Can you work these out from the model? Positions are in its coordinate system, mm. A direction names the side the tool comes from. Coordinates: 2 decimals unless noted, no trailing zeros. Loops run counter-clockwise (first coordinate to the right, second up) from the corner with the lowest first, then second, coordinate; pieces in that order, holes last.
Autodesk Inventor part; units mm, degrees
ref_plane "YZ Plane" through (0, 0, 0) normal (1, 0, 0) x (0, 1, 0)
ref_plane "XZ Plane" through (0, 0, 0) normal (0, 1, 0) x (-1, 0, 0)
ref_plane "XY Plane" through (0, 0, 0) normal (0, 0, 1) x (1, 0, 0)
sketch "スケッチ1" plane through (0, 0, 0) normal (0, 0, 1) x (1, 0, 0)
  line L0 (-12, -6) -> (12, -6)
  line L1 (12, -6) -> (12, 6)
  line L2 (12, 6) -> (-12, 6)
  line L3 (-12, 6) -> (-12, -6)
  line L4 (-12, -6) -> (12, 6) construction
  line L5 (12, -6) -> (-12, 6) construction
  point P0 (0, 0)
  dimension "d0" = 24
  dimension "d1" = 12
extrude "押し出し1" add sketch "スケッチ1" against normal blind 26.7
sketch "スケッチ2" plane through (0, 0, 0) normal (0, 0, 1) x (1, 0, 0)
  line L0 (-15, 0) -> (15, 0) construction
  line L1 (-15, -4) -> (15, -4)
  line L2 (15, 4) -> (-15, 4)
  arc A0 (-15, 4) -> (-15, -4) centre (-15, 0) ccw
  arc A1 (15, -4) -> (15, 4) centre (15, 0) ccw
  point P0 (0, 0)
  dimension "d4" = 30
  dimension "d5" = 4
extrude "押し出し2" add sketch "スケッチ2" against normal blind 7
sketch "スケッチ3" plane through (0, 0, 0) normal (0, 0, 1) x (1, 0, 0)
  arc A0 (-15, 4) -> (-15, -4) centre (-15, 0) ccw
  arc A1 (15, -4) -> (15, 4) centre (15, 0) ccw
  point P0 (0, 0)
hole "穴1" at (15, 0, 0) at (-15, 0, 0) direction (0, 0, -1) diameter 2.459 end through all
sketch "スケッチ4" plane through (0, 0, -26.7) normal (0, 0, -1) x (-1, 0, 0)
  circle A0 centre (0, 0) radius 5.5
  line L0 (12, 6) -> (-12, 6)
  dimension "d30" = 11
extrude "押し出し3" add sketch "スケッチ4" along normal blind 2.8
sketch "スケッチ5" plane through (-12, 6, 0) normal (0, 1, 0) x (1, 0, 0)
  line L0 (17.5, 29.5) -> (6.5, 29.5)
  line L1 (6.5, 26.7) -> (17.5, 26.7)
  line L2 (6.5, 26.7) -> (17.5, 26.7)
  line L3 (6.5, 26.7) -> (6.5, 26.7)
  line L4 (17.5, 26.7) -> (24, 15)
  line L5 (24, 0) -> (24, 26.7)
  line L6 (24, 0) -> (0, 0)
  line L7 (6.5, 26.7) -> (0, 15)
  line L8 (0, 0) -> (0, 26.7)
  line L9 (24, 0) -> (0, 0)
  line L10 (24, 0) -> (24, 26.7)
  line L11 (0, 26.7) -> (24, 26.7)
  line L12 (0, 0) -> (0, 26.7)
  point P0 (12, 0)
  point P1 (17.5, 26.7)
  point P2 (6.5, 26.7)
  dimension "d18" = 15
  dimension "d19" = 15
extrude "押し出し4" cut sketch "スケッチ5" against normal through all contours L7 L8 L11 | L11 L5 L4
sketch "スケッチ6" plane through (0, 0, 0) normal (0, 0, 1) x (1, 0, 0)
  line L0 (-8.65, -6) -> (8.65, -6)
  line L1 (8.65, -6) -> (8.65, 6)
  line L2 (8.65, 6) -> (-8.65, 6)
  line L3 (-8.65, 6) -> (-8.65, -6)
  line L4 (-8.65, -6) -> (8.65, 6) construction
  line L5 (8.65, -6) -> (-8.65, 6) construction
  line L6 (12, 6) -> (-12, 6)
  point P0 (0, 0)
  dimension "d22" = 17.3
extrude "押し出し5" cut sketch "スケッチ6" against normal blind 10
sketch "スケッチ7" plane through (0, 0, -10) normal (0, 0, 1) x (1, 0, 0)
  line L0 (-5, -5) -> (5, -5)
  line L1 (5, -5) -> (5, 5)
  line L2 (5, 5) -> (-5, 5)
  line L3 (-5, 5) -> (-5, -5)
  line L4 (-5, -5) -> (5, 5) construction
  line L5 (5, -5) -> (-5, 5) construction
  point P0 (0, 0)
  dimension "d25" = 10
  dimension "d26" = 10
extrude "押し出し6" add sketch "スケッチ7" along normal blind 10
fillet "フィレット1" radius 1 14 edges at (12, 4, -3.5) (12, -4, -3.5) (-12, -4, -3.5) (-12, -6, -7.5) (12, -6, -7.5) (12, 6, -7.5) (-12, 4, -3.5) (-12, 6, -7.5) (-8.75, 6, -20.85) (-12, 0, -15) (-8.75, -6, -20.85) (8.75, -6, -20.85) (12, 0, -15) (8.75, 6, -20.85)
properties part number "USB2-MBMPAF-XXE" material "ABS プラスチック"
Item 1: I'm going to push flat-ended pins straight in: P1, Ø0.6, axis at x = 13.5, z = -2.5, coming from the -Y side; P2, Ø1, axis at x = -13.5, z = -2.5, coming from the +Y side; P3, Ø2, axis at y = -4.5, z = -13.5, coming from the +X side. Where does each tip first touch, or does it pass through?
Results are:
P1: stops at y = -4
P2: stops at y = 4
P3: stops at x = 12
Item 2: On a 3-axis mill with a long thin cutter (end or side, diameter ignored), from which of +Z, -Z, +X, -X, +Y, -Y can I reach the whole of each face in a straight line? I mean faces 1 (the face through (-8.243, -5.715, -21.144)), 2 (the face through (16, 1, -7)), 3 (the face through (-16, 1, -7)), 4 (the face through (0, 5.7, -26.7)), 5 (the face through (-5, 0, -5)). Say none if no direction works.
Results are:
face 1: -Z, -X, -Y
face 2: -Z, +X, +Y, -Y
face 3: -Z, -X, +Y, -Y
face 4: -Z, +Y
face 5: +Z, +Y, -Y
Item 3: Suppose I cut it at A-A, the plane z = -11.75. Please give me the cut outline in (x, y), plus the area to 3 significant figures.
Results are:
outline: (-12, -5) arc R1 ccw to (-11, -6) - (11, -6) arc R1 ccw to (12, -5) - (12, 5) arc R1 ccw to (11, 6) - (-11, 6) arc R1 ccw to (-12, 5) - close
area: 287 mm2
Item 4: Suppose I cut it at B-B, the plane x = 0. Please give me the cut outline in (y, z).
Results are:
outline: (-6, -26.7) - (-5.5, -26.7) - (-5.5, -29.5) - (5.5, -29.5) - (5.5, -26.7) - (6, -26.7) - (6, -10) - (5, -10) - (5, 0) - (-5, 0) - (-5, -10) - (-6, -10) - close
Item 5: We'd pull the mould along X, two halves only. Please class faces 6 (the face through (-16.22, 0.16, -3.55)), 7 (the face through (14, 4, -3)), 8 (the face through (12.285, -4.301, -3.549)): +X half, -X half, draft (parallel to the pull), parting line (faces both ways), or undercut.
Results are:
face 6: undercut
face 7: draft
face 8: +X half
Item 6: I need wall thicknesses on line 1 along X through (y, z) = (0, -1.25); line 2 along Y through (x, z) = (-15, -3.25); line 3 along X through (y, z) = (-1.5, -8.75). Which ranges of each line are inside material? Lowest first, please.
Results are:
line 1: x = -19 to -16.23, -13.77 to -8.65, -5 to 5, 8.65 to 13.77, 16.23 to 19
line 2: y = -4 to -1.23, 1.23 to 4
line 3: x = -12 to -8.65, -5 to 5, 8.65 to 12
